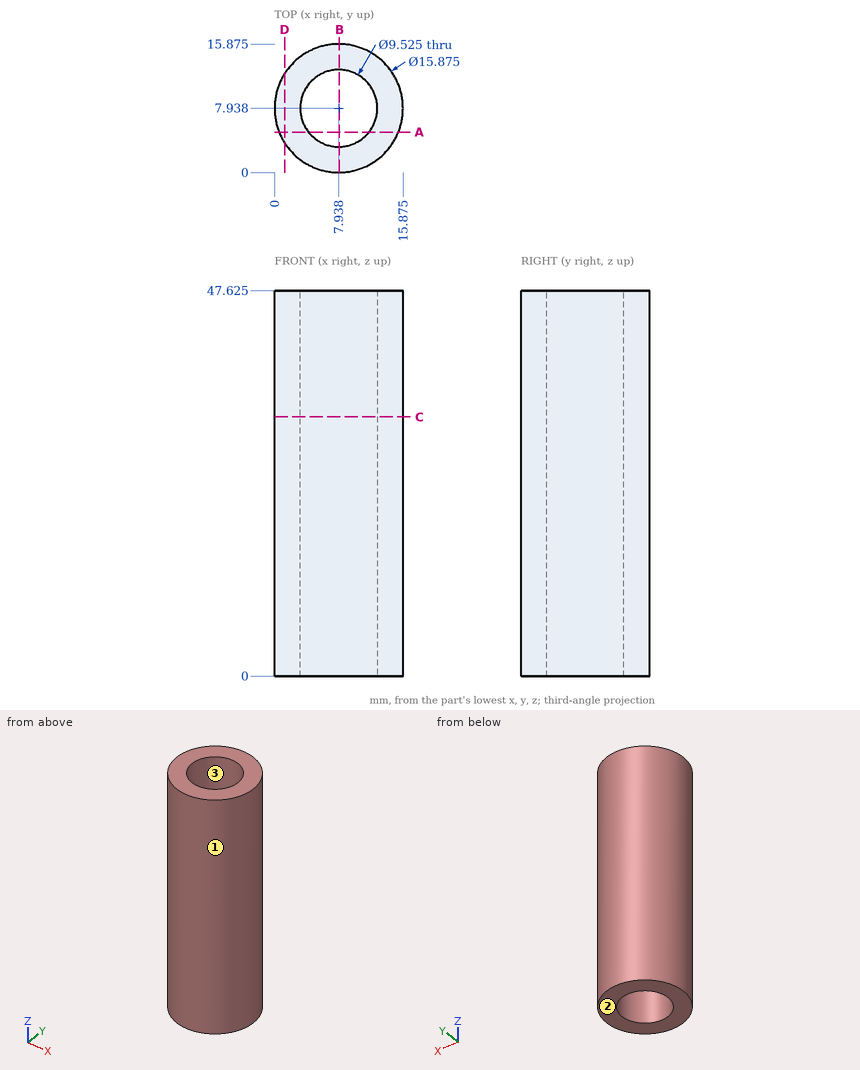
For this review, use the dimensioned drawing (mm, ordinates from the lowest corner) and the shaded views. Round coordinates to 2 decimals unless told otherwise and drop trailing zeros. Write each loop counter-clockwise with the first axis right and the second up, starting at its lowest first coordinate (ties: lowest second). Pieces come first, ordered by that corner, then holes. Notation, with made-up numbers: (-10.75, 23.5) - (41.25, 23.5) arc R18 ccw to (41.25, 27.5) - close; hole circle Ø2 at (-28.5, 49). An arc over 180 degrees is marked (long way). Use a Markdown table: item, result.
Q1. Wall thickness on line 1 along Y through (x, z) = (8, 12) (1 decimal); line 2 along Y through (x, z) = (12.25, 2) (1 decimal): over which ranges is each line inside the solid? List them lowest first.
Derived:
| item | result |
|---|---|
| line 1 | y = 0 to 3.2, 12.7 to 15.9 |
| line 2 | y = 1.3 to 5.9, 10 to 14.6 |
Q2. We need section D-D (x = 1.25). Give the boundary of the cut face in (y, z) (1 decimal).
Derived:
| item | result |
|---|---|
| outline | (3.7, 0) - (12.2, 0) - (12.2, 47.6) - (3.7, 47.6) - close |
Q3. We need section C-C (z = 32). Give the boundary of the cut face in (x, y) (1 decimal), plus the area to 3 significant figures.
Derived:
| item | result |
|---|---|
| outline | circle Ø15.9 at (7.9, 7.9); hole circle Ø9.5 at (7.9, 7.9) |
| area | 127 mm2 |
Q4. We need section B-B (x = 8). Give the boundary of the cut face in (y, z) (1 decimal).
Derived:
| item | result |
|---|---|
| outline | (0, 0) - (3.2, 0) - (3.2, 47.6) - (0, 47.6) - close; (12.7, 0) - (15.9, 0) - (15.9, 47.6) - (12.7, 47.6) - close |
Q5. The part is to be moulded in two halves that separate along X. For the marked faces 1, 2 and 3, say which applies: pulls with the +X half, pulls with the -X half, needs draft (parallel to the pull), parting line crosses it, or undercut.
Derived:
| item | result |
|---|---|
| face 1 | parting line crosses it |
| face 2 | needs draft |
| face 3 | undercut |
Q6. Clearance check with flat-ended pins moving along their axes: pin 1 (8 mm diameter, centred on x = 3, z = 15.5, fed in from +Y); pin 2 (4 mm diameter, centred on y = 11, z = 39, fed in from -X). State where each tip first meets the part, or that it passes through.
Derived:
| item | result |
|---|---|
| pin 1 | stops at y = 15.82 |
| pin 2 | stops at x = 0.07 |
Q7. We need section A-A (y = 5). Give the boundary of the cut face in (x, z) (1 decimal).
Derived:
| item | result |
|---|---|
| outline | (0.6, 0) - (4.2, 0) - (4.2, 47.6) - (0.6, 47.6) - close; (11.7, 0) - (15.3, 0) - (15.3, 47.6) - (11.7, 47.6) - close |
